Check sheet for the modelled part. Datum: model origin and axes. Units: mm. A direction names the side the tool comes from. Give positions to 0.01 mm unless a question says otherwise; leave off trailing zeros. Loops run counter-clockwise (first coordinate to the right, second up) from the corner with the lowest first, then second, coordinate; pieces in that order, holes last. Notation, with made-up numbers: (-37, 67.25) - (12, 67.25) arc R19 ccw to (12, 103.25) - close; hole circle Ø9 at (-6.75, 57.25). An arc over 180 degrees is marked (long way). Use one line per item in the form item = value.
from build123d import *

# Parameters (mm, degrees)
F0_R     = 7
F0_R_2   = 1.5
F0_R_3   = 3
F1_DEPTH = 2
F2_DEPTH = 14
F3_R     = 2.05
F4_DEPTH = 14


# Not quite as in the source:
# - a feature names something its author has since deleted; it is built from what else it names


with BuildPart() as f1:
    # F0 (on Front) → F1 (new body)
    with BuildSketch(Plane.XZ):
        Circle(F0_R)
        with Locations((-4.6, 0)):
            Circle(F0_R_2, mode=Mode.SUBTRACT)
        Circle(F0_R_3, mode=Mode.SUBTRACT)
        with Locations((4.6, 0)):
            Circle(F0_R_2, mode=Mode.SUBTRACT)
        Circle(F0_R_3)
    extrude(amount=F1_DEPTH)

    # F0 (on Front) → F2 (join)
    with BuildSketch(Plane.XZ):
        Circle(F0_R_3)
    extrude(amount=-F2_DEPTH)

    # F3 (on face) → F4 (cut)
    with BuildSketch(Plane(origin=(0, 14, 0), x_dir=(-1, 0, 0), z_dir=(0, 1, 0))):
        Circle(F3_R)
    extrude(amount=-F4_DEPTH, mode=Mode.SUBTRACT)


solid = f1.part
Item 1: Thickness scan on L1, parallel to Z at x = 0, y = 10.5; L2, parallel to Y at x = 5, z = 4.5; L3, parallel to X at y = 3.5, z = 1.75. Record the ranges inside material, lowest first.
Answer block:
L1 = -3 to -2.05, 2.05 to 3
L2 = -2 to 0
L3 = -2.44 to -1.07, 1.07 to 2.44
Item 2: Gauge pin test, flat ends, axial feed: P1, Ø3.5, axis at x = -4.6, z = 0, coming from the -Y side; P2, Ø2, axis at x = 0.5, z = 0, coming from the +Y side; P3, Ø4, axis at x = -4.5, y = 6.5, coming from the -Z side; P4, Ø6, axis at x = -4.5, y = 5.5, coming from the +Z side. Record the tip position at first contact, or that the pin passes through.
Answer block:
P1 = -2
P2 = 0
P3 = -1.66
P4 = 2.6
Item 3: Section check A-A on z = 0. Record the boundary of the cut face in (x, y), then the cut area to 3 significant figures.
Answer block:
outline = (-7, -2) - (-6.1, -2) - (-6.1, 0) - (-7, 0) - close; (-3.1, -2) - (3.1, -2) - (3.1, 0) - (3, 0) - (3, 14) - (2.05, 14) - (2.05, 0) - (-2.05, 0) - (-2.05, 14) - (-3, 14) - (-3, 0) - (-3.1, 0) - close; (6.1, -2) - (7, -2) - (7, 0) - (6.1, 0) - close
area = 42.6 mm2
Item 4: Section check B-B on x = -3.5. Record the boundary of the cut face in (y, z), then the cut area to 3 significant figures.
Answer block:
outline = (-2, -6.06) - (0, -6.06) - (0, -1.02) - (-2, -1.02) - close; (-2, 1.02) - (0, 1.02) - (0, 6.06) - (-2, 6.06) - close
area = 20.2 mm2
Item 5: Mould release check, pull along Z, two halves, no side actions. Record for faces 1 (the face through (-3.214, -0.986, -0.575)), 2 (the face through (0, -2, 0)), 3 (the face through (-3, 7, 0)), 4 (the face through (0.267, 7.098, 2.033)): released by +Z, released by -Z, zero draft, split by the parting line, or undercut.
Answer block:
face_1 = undercut
face_2 = zero draft
face_3 = split by the parting line
face_4 = undercut
Item 6: Section check C-C on x = 4.6. Record the boundary of the cut face in (y, z).
Answer block:
outline = (-2, -5.28) - (0, -5.28) - (0, -1.5) - (-2, -1.5) - close; (-2, 1.5) - (0, 1.5) - (0, 5.28) - (-2, 5.28) - close
Item 7: Access from +Z, -Z, +X, -X, +Y, -Y to the whole of each face (thin tool, end or side, straight path). Record for faces 5 (the face through (6.466, -0.986, -2.681)), 6 (the face through (0, 0, 0)).
Answer block:
face_5 = +Y, -Y
face_6 = +Y
Item 8: Section check D-D on y = 10.25. Record the boundary of the cut face in (x, z), then the cut area to 3 significant figures.
Answer block:
outline = circle Ø6 at (0, 0); hole circle Ø4.1 at (0, 0)
area = 15.1 mm2
